Autodesk Inventor part; units mm, degrees
ref_plane "YZ Plane" through (0, 0, 0) normal (1, 0, 0) x (0, 1, 0)
ref_plane "XZ Plane" through (0, 0, 0) normal (0, 1, 0) x (-1, 0, 0)
ref_plane "XY Plane" through (0, 0, 0) normal (0, 0, 1) x (1, 0, 0)
sketch "Skizze1" plane through (0, 0, 0) normal (0, 1, 0) x (-1, 0, 0)
  line L0 (0, 0) -> (4.32, 0)
  line L1 (4.32, 0) -> (4.32, -3.81)
  line L2 (4.32, -3.81) -> (12.7, -3.81)
  line L3 (12.7, -3.81) -> (12.7, -16)
  line L4 (12.7, -16) -> (4.32, -16)
  line L5 (4.32, -16) -> (4.32, -19.81)
  line L6 (4.32, -19.81) -> (0, -19.81)
  line L7 (0, -19.81) -> (0, 0)
  line L8 (2.16, 0) -> (2.16, -2.16)
  line L9 (2.16, -19.81) -> (2.16, -17.65)
  circle A0 centre (2.16, -2.16) radius 1.22
  circle A1 centre (2.16, -17.65) radius 1.22
  dimension "d0" = 4.32
  dimension "d1" = 3.81
  dimension "d2" = 8.38
  dimension "d3" = 12.19
  dimension "d4" = 3.81
  dimension "d5" = 2.16
  dimension "d6" = 2.16
  dimension "d7" = 2.44
  dimension "d8" = 2.44
extrude "Extrusion1" add sketch "Skizze1" along normal blind 5.08
properties part number "OPB732" material "LCP-Kunststoff"
Could you check a few things on this model? Use its own coordinates, in mm. A direction names the side the tool comes from. Round coordinates to 2 decimals unless told otherwise and drop trailing zeros. Loops run counter-clockwise (first coordinate to the right, second up) from the corner with the lowest first, then second, coordinate; pieces in that order, holes last.
Q1. On a 3-axis mill with a long thin cutter (end or side, diameter ignored), from which of +Z, -Z, +X, -X, +Y, -Y can I reach the whole of each face in a straight line? I mean faces 4 (the flat face through (-4.32, 3, -2)), 5 (the flat face through (-2, 3, 0)), 6 (the flat face through (-9, 3, -16)). Say none if no direction works.
Q2. Thinking about a two-plate mould opening in Z: for faces 1 (the flat face through (-6, 5.08, -10)), 2 (the flat face through (-2, 3, -19.81)), 3 (the cylindrical face through (-2.723, 2.504, -16.568)), which applies, pulls with the +Z half, pulls with the -Z half, needs draft (parallel to the pull), parting line crosses it, or undercut?
Q3. For P1, Ø3, axis at x = -2.16, z = -2.16, coming from the +Y side; P2, Ø1.1, axis at y = 3, z = -18.5, coming from the -X side; P3, Ø2.5, axis at x = -10, y = 3, coming from the +Z side, each with a flat end and sliding along its axis, tell me the tip position at first contact or that it passes through.
Q4. I want a section at C-C (y = 1.9). Write out the boundary of the cut face in (x, z), and give its area (3 significant figures).
Q5. Please list where these lines run through material, in increasing order: L1, parallel to X at y = 2.7, z = -17.65; L2, parallel to Z at x = -2.16, y = 1.7; L3, parallel to Z at x = -7, y = 3.7.
Q6. I want a section at D-D (x = -6.5). Write out the boundary of the cut face in (y, z).
Q7. I want a section at A-A (z = -2.16). Write out the boundary of the cut face in (x, y).
Q8. I want a section at B-B (x = -2.16). Write out the boundary of the cut face in (y, z).
Answer below:
1. face 4: +Z, -X, +Y, -Y
1. face 5: +Z, +X, -X, +Y, -Y
1. face 6: -Z, -X, +Y, -Y
2. face 1: needs draft
2. face 2: pulls with the -Z half
2. face 3: undercut
3. P1: stops at y = 5.08
3. P2: stops at x = -4.32
3. P3: stops at z = -3.81
4. outline: (-12.7, -16) - (-4.32, -16) - (-4.32, -19.81) - (0, -19.81) - (0, 0) - (-4.32, 0) - (-4.32, -3.81) - (-12.7, -3.81) - close; hole circle Ø2.44 at (-2.16, -17.65); hole circle Ø2.44 at (-2.16, -2.16)
4. area: 178 mm2
5. L1: x = -4.32 to -3.38, -0.94 to 0
5. L2: z = -19.81 to -18.87, -16.43 to -3.38, -0.94 to 0
5. L3: z = -16 to -3.81
6. outline: (0, -16) - (5.08, -16) - (5.08, -3.81) - (0, -3.81) - close
7. outline: (-4.32, 0) - (-3.38, 0) - (-3.38, 5.08) - (-4.32, 5.08) - close; (-0.94, 0) - (0, 0) - (0, 5.08) - (-0.94, 5.08) - close
8. outline: (0, -19.81) - (5.08, -19.81) - (5.08, -18.87) - (0, -18.87) - close; (0, -16.43) - (5.08, -16.43) - (5.08, -3.38) - (0, -3.38) - close; (0, -0.94) - (5.08, -0.94) - (5.08, 0) - (0, 0) - close
